from build123d import *

# Parameters (mm, degrees)
BOSS_EXTRUDE1_DEPTH = 15
FILLET1_R           = 7.5
SKETCH2_R           = 2.5
CUT_EXTRUDE1_DEPTH  = 40.023610486


with BuildPart() as part:
    # Sketch1 → Boss-Extrude1 (new body)
    with BuildSketch(Plane(origin=(0, 0, 0), x_dir=(1, 0, 0), z_dir=(0, 1, 0))):
        with BuildLine():
            Line((-2.5, 15.676913759), (-2.5, 35.676913759))
            Line((-2.5, 35.676913759), (2.5, 35.676913759))
            Line((2.5, 35.676913759), (2.5, 15.676913759))
            ThreePointArc((2.5, 15.676913759), (0, 15.875), (-2.5, 15.676913759))
        make_face()
    extrude(amount=BOSS_EXTRUDE1_DEPTH)

    # Fillet1
    fillet1_edges = [part.edges().sort_by_distance(p)[0] for p in [
        (0, 0, -35.676913759),
        (0, 15, -35.676913759),
    ]]
    fillet(fillet1_edges, radius=FILLET1_R - 0.0001)  # a hair under: the kernel refuses the full size

    # Sketch2 → Cut-Extrude1 (cut, through all)
    with BuildSketch(Plane.ZY.offset(2.5)):
        with Locations((-28.176913759, 7.5)):
            Circle(SKETCH2_R)
    extrude(amount=-CUT_EXTRUDE1_DEPTH, mode=Mode.SUBTRACT)


solid = part.part
Can you work these out from the model? Positions are in its coordinate system, mm. Coordinates: 2 decimals unless noted, no trailing zeros. Loops run counter-clockwise (first coordinate to the right, second up) from the corner with the lowest first, then second, coordinate; pieces in that order, holes last. Notation, with made-up numbers: (32.5, 30) - (79.5, 30) arc R29 ccw to (79.5, 54) - close; hole circle Ø10 at (70.25, -2.75). An arc over 180 degrees is marked (long way). Answer as a JSON object with one key per item and string values. Group by question number.
Item 1: If we section it at D-D (y = 13): List the corners of the cut face in (x, z) for me (3 decimals).
Item 2: For pin 1 (3 mm diameter, centred on x = 2, y = 6.5, fed in from +Z); pin 2 (1.5 mm diameter, centred on x = 1, y = 4.5, fed in from -Z), each with a flat end and sliding along its axis, tell me the tip position at first contact or that it passes through.
Item 3: If we mould it in two halves opening along X, with no side actions, what happens to faces 1 (the face through (0.035, 7.395, -15.875)), 2 (the face through (-2.5, 7.4, -25.5)), 3 (the face through (2.5, 7, -24)), 4 (the face through (0.035, 2.255, -33.538))? For each: released by +X, released by -X, zero draft, split by the parting line, or undercut.
Item 4: If I drill on L1, parallel to Y at x = 0.7, z = -29.75; L2, parallel to Z at x = 0.5, y = 9.25; L3, parallel to Y at x = 1.9, z = -30, over which ranges is the centre line in solid material (lowest first)? Write a range as from..to.
Item 5: If we section it at A-A (y = 6.5): List the corners of the cut face in (x, z) for me (3 decimals).
Returned:
{
 "1": {"outline": "(-2.5, -33.276) - (2.5, -33.276) - (2.5, -15.677) arc R15.875 cw to (-2.5, -15.677) - close"},
 "2": {"pin 1": "stops at z = -15.68", "pin 2": "stops at z = -35.33"},
 "3": {"face 1": "undercut", "face 2": "released by -X", "face 3": "released by +X", "face 4": "zero draft"},
 "4": {"L1": "y = 0.17..5.56, 9.44..14.83", "L2": "z = -35.47..-29.96, -26.39..-15.87", "L3": "y = 0.22..5.79, 9.21..14.78"},
 "5": {"outline": "(-2.5, -35.61) - (2.5, -35.61) - (2.5, -30.468) - (-2.5, -30.468) - close; (-2.5, -25.886) - (2.5, -25.886) - (2.5, -15.677) arc R15.875 cw to (-2.5, -15.677) - close"}
}
